Build history of the part. All positions in model axes, mm. Face numbers are marked on the shaded views. A direction names the side the tool comes from. Give positions to 0.01 mm unless a question says otherwise; leave off trailing zeros. Loops run counter-clockwise (first coordinate to the right, second up) from the corner with the lowest first, then second, coordinate; pieces in that order, holes last. Notation, with made-up numbers: (23, 67.25) - (51, 67.25) arc R5 ccw to (51, 75.25) - close; hole circle Ø9 at (-5.75, -37.75). An arc over 180 degrees is marked (long way). Return JSON: item names as keys, results as strings. Group by question number.
1) Slice it at C-C (y = -31.5). List the corners of the cut face in (x, z), and give its area (3 significant figures).
2) Drop flat-ended pins along their axis: pin 1 (6 mm diameter, centred on y = 1.5, z = -58.5, fed in from +X); pin 2 (4 mm diameter, centred on x = 25.88, z = -96.59, fed in from +Y); pin 3 (4 mm diameter, centred on x = -9, y = 50.5, fed in from -Z). Give the stop position or say it passes through.
3) 3-axis set-ups, long thin cutter, end or side, ignore diameter. For the marked faces 1, 2 and 3: which of +Z, -Z, +X, -X, +Y, -Y reach the whole face in a straight line?
4) Drill centre lines: probe 1 along Y at (x, z) = (-102, -10.5); probe 2 along X at (y, z) = (19, -10); probe 3 along Y at (x, z) = (-52.5, -60). Where is each one in solid material? Low to high. Write a range as from..to.
5) Slice it at B-B (x = 0). List the corners of the cut face in (y, z).
6) Slice it at A-A (y = 19.8). List the corners of the cut face in (x, z).
7) Slice it at D-D (y = 68.5). List the corners of the cut face in (x, z).
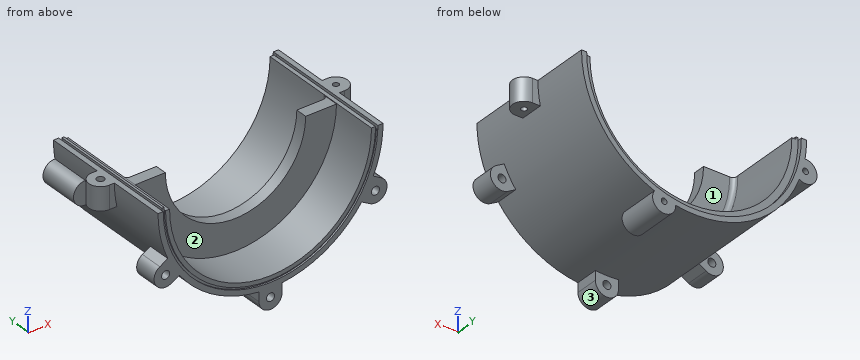
```python
from build123d import *

# Parameters (mm, degrees)
REVOLU_O2_ANGLE            = 180
ESBO_O4_R                  = 10
RESSALTO_EXTRUS_O1_DEPTH   = 35
RESSALTO_EXTRUS_O2_DEPTH   = 20
ESBO_O8_R                  = 3.5
CORTE_EXTRUS_O2_DEPTH      = 20
PADR_OCIRCULAR1_COUNT      = 6
ESBO_O6_R                  = 2.5
CORTE_EXTRUS_O1_DEPTH      = 15
ESBO_O10_W                 = 2.2
ESBO_O10_H                 = 116.4
CORTE_EXTRUS_O4_DEPTH      = 3.5
ESBO_O11_W                 = 2
ESBO_O11_H                 = 114.9
RESSALTO_EXTRUS_O5_DEPTH   = 2
ESBO_O12_R                 = 3.25
RESSALTO_EXTRUS_O6_DEPTH   = 20
ESBO_O13_R                 = 2.5
RESSALTO_EXTRUS_O7_DEPTH   = 20
ESBO_O16_R                 = 93
CORTE_EXTRUS_O6_DEPTH      = 10
ESBO_O17_R                 = 92.967356783
ESBO_O17_R_2               = 90.967356783
CORTE_EXTRUS_O7_DEPTH      = 1.5
CORTE_EXTRUS_O9_DEPTH      = 41.2
CORTE_EXTRUS_O9_DEPTH_BACK = 80.8


with BuildPart() as part:
    # Esboço3 → Revolução2 (revolve)
    with BuildSketch(Plane.XY):
        with BuildLine():
            Line((97.5, 79.8), (97.5, 11.304491341))
            Line((97.5, 11.304491341), (97.5, 0))
            Line((97.5, 0), (97.5, -40.2))
            Line((97.5, -40.2), (87.5, -40.2))
            Line((87.5, -40.2), (87.5, 0))
            Line((87.5, 0), (60.342408243, 0))
            Line((60.342408243, 0), (60.342408243, 10.2))
            Line((60.342408243, 10.2), (83.5, 10.2))
            ThreePointArc((83.5, 10.2), (86.328427125, 11.371572875), (87.5, 14.2))
            Line((87.5, 14.2), (87.5, 76.2))
            Line((87.5, 76.2), (93, 76.2))
            Line((93, 76.2), (93, 79.8))
            Line((93, 79.8), (97.5, 79.8))
        make_face()
    revolve(axis=Axis((0, -3.322055656, 0), (0, 1, 0)), revolution_arc=REVOLU_O2_ANGLE)

    # Esboço4 → Ressalto-extrusão1 (add)
    with BuildSketch(Plane(origin=(0, 79.8, 0), x_dir=(1, 0, 0), z_dir=(0, 1, 0))):
        with Locations((25.881656302, 96.591656302)):
            Circle(ESBO_O4_R)
        with Locations((-96.591656302, 25.881656302)):
            Circle(ESBO_O4_R)
    extrude(amount=-RESSALTO_EXTRUS_O1_DEPTH)

    # Esboço5 → Ressalto-extrusão2 (add)
    with BuildSketch(Plane.XZ.offset(40.2)):
        with BuildLine():
            Line((10, -105), (10, -96.985823706))
            Line((10, -96.985823706), (-10, -96.985823706))
            Line((-10, -96.985823706), (-10, -105))
            ThreePointArc((-10, -105), (0, -115), (10, -105))
        make_face()
    ressalto_extrus_o2 = extrude(amount=-RESSALTO_EXTRUS_O2_DEPTH)

    # Esboço8 → Corte-extrusão2 (cut)
    with BuildSketch(Plane.XZ.offset(40.2)):
        with Locations((0, -105)):
            Circle(ESBO_O8_R)
    corte_extrus_o2 = extrude(amount=-CORTE_EXTRUS_O2_DEPTH, mode=Mode.SUBTRACT)

    # PadrãoCircular1: Ressalto-extrusão2, Corte-extrusão2 ×6 about axis, 3 skipped
    padr_ocircular1_axis = Axis((0, 0, 0), (0, 1, 0))
    add([ressalto_extrus_o2.rotate(padr_ocircular1_axis, i * 360 / PADR_OCIRCULAR1_COUNT) for i in range(1, PADR_OCIRCULAR1_COUNT) if i not in (2, 3, 4)])
    add([corte_extrus_o2.rotate(padr_ocircular1_axis, i * 360 / PADR_OCIRCULAR1_COUNT) for i in range(1, PADR_OCIRCULAR1_COUNT) if i not in (2, 3, 4)], mode=Mode.SUBTRACT)

    # Esboço6 → Corte-extrusão1 (cut)
    with BuildSketch(Plane(origin=(0, 79.8, 0), x_dir=(1, 0, 0), z_dir=(0, 1, 0))):
        with Locations((25.881656302, 96.591656302)):
            Circle(ESBO_O6_R)
        with Locations((-96.591656302, 25.881656302)):
            Circle(ESBO_O6_R)
    extrude(amount=-CORTE_EXTRUS_O1_DEPTH, mode=Mode.SUBTRACT)

    # Esboço10 → Corte-extrusão4 (cut)
    with BuildSketch(Plane.XY):
        with Locations((92, 18)):
            Rectangle(ESBO_O10_W, ESBO_O10_H)
    extrude(amount=-CORTE_EXTRUS_O4_DEPTH, mode=Mode.SUBTRACT)

    # Esboço11 → Ressalto-extrusão5 (add)
    with BuildSketch(Plane.XY):
        with Locations((-92, 18.75)):
            Rectangle(ESBO_O11_W, ESBO_O11_H)
    extrude(amount=RESSALTO_EXTRUS_O5_DEPTH)

    # Esboço12 → Ressalto-extrusão6 (add)
    with BuildSketch(Plane.XY):
        with BuildLine():
            Line((-102, 29.8), (-87.5, 29.8))
            Line((-87.5, 29.8), (-87.5, 9.8))
            Line((-87.5, 9.8), (-102, 9.8))
            ThreePointArc((-102, 9.8), (-112, 19.8), (-102, 29.8))
        make_face()
        with Locations((-102, 19.8)):
            Circle(ESBO_O12_R, mode=Mode.SUBTRACT)
    extrude(amount=-RESSALTO_EXTRUS_O6_DEPTH)

    # Esboço13 → Ressalto-extrusão7 (add)
    with BuildSketch(Plane.XY):
        with BuildLine():
            Line((102, 29.8), (93.1, 29.8))
            Line((93.1, 29.8), (93.1, 9.8))
            Line((93.1, 9.8), (102, 9.8))
            ThreePointArc((102, 9.8), (112, 19.8), (102, 29.8))
        make_face()
        with Locations((102, 19.8)):
            Circle(ESBO_O13_R, mode=Mode.SUBTRACT)
    extrude(amount=-RESSALTO_EXTRUS_O7_DEPTH)

    # Esboço16 → Corte-extrusão6 (cut)
    with BuildSketch(Plane(origin=(0, 76.2, 0), x_dir=(1, 0, 0), z_dir=(0, 1, 0))):
        Circle(ESBO_O16_R)
    extrude(amount=CORTE_EXTRUS_O6_DEPTH, mode=Mode.SUBTRACT)

    # Esboço17 → Corte-extrusão7 (cut)
    with BuildSketch(Plane.XZ.offset(40.2)):
        Circle(ESBO_O17_R)
        Circle(ESBO_O17_R_2, mode=Mode.SUBTRACT)
    extrude(amount=-CORTE_EXTRUS_O7_DEPTH, mode=Mode.SUBTRACT)

    # Esboço21 → Corte-extrusão9 (cut, two sides)
    with BuildSketch(Plane.XZ) as corte_extrus_o9_sk:
        with BuildLine():
            Line((-87.5, 0), (87.5, 0))
            ThreePointArc((87.5, 0), (87.499642853, -0.25000102), (87.498571417, -0.5))
            Line((87.498571417, -0.5), (60.84035372, -0.5))
            ThreePointArc((60.84035372, -0.5), (0, -60.842408243), (-60.84035372, -0.5))
            Line((-60.84035372, -0.5), (-87.498571417, -0.5))
            ThreePointArc((-87.498571417, -0.5), (-87.499642853, -0.25000102), (-87.5, 0))
        make_face()
    extrude(amount=CORTE_EXTRUS_O9_DEPTH, mode=Mode.SUBTRACT)
    extrude(corte_extrus_o9_sk.sketch, amount=-CORTE_EXTRUS_O9_DEPTH_BACK, mode=Mode.SUBTRACT)


solid = part.part
```
Results:
{
 "1": {"outline": "(-97.5, 0) arc R97.5 ccw to (-88.99, -39.83) - (-95.93, -43.84) arc R10 ccw to (-85.93, -61.16) - (-78.99, -57.15) arc R97.5 ccw to (-10, -96.99) - (-10, -105) arc R10 ccw to (10, -105) - (10, -96.99) arc R97.5 ccw to (78.99, -57.15) - (85.93, -61.16) arc R10 ccw to (95.93, -43.84) - (88.99, -39.83) arc R97.5 ccw to (97.5, 0) - (93.1, 0) - (93.1, -3.5) - (90.9, -3.5) - (90.9, 0) - (87.5, 0) arc R87.5 cw to (-87.5, 0) - (-91, 0) - (-91, 2) - (-93, 2) - (-93, 0) - close; hole circle Ø7 at (-90.93, -52.5); hole circle Ø7 at (0, -105); hole circle Ø7 at (90.93, -52.5)", "area": "3,720 mm2"},
 "2": {"pin 1": "x = 80.16", "pin 2": "y = 64.8", "pin 3": "z = -97.25"},
 "3": {"face 1": "+Z, +Y", "face 2": "+Z, -Y", "face 3": "-Z, +Y, -Y"},
 "4": {"probe 1": "9.8..16.55, 23.05..29.8", "probe 2": "-111.97..-105.15, -98.85..-86.93, 86.93..99.63, 104.37..111.97", "probe 3": "0..10.2"},
 "5": {"outline": "(-40.2, -115) - (-20.2, -115) - (-20.2, -108.5) - (-40.2, -108.5) - close; (-40.2, -101.5) - (-20.2, -101.5) - (-20.2, -97.5) - (79.8, -97.5) - (79.8, -93) - (76.2, -93) - (76.2, -87.5) - (14.2, -87.5) arc R4 cw to (10.2, -83.5) - (10.2, -60.84) - (0, -60.84) - (0, -87.5) - (-40.2, -87.5) - (-40.2, -90.97) - (-38.7, -90.97) - (-38.7, -92.97) - (-40.2, -92.97) - close"},
 "6": {"outline": "(-112, -20) - (-105.25, -20) - (-105.25, 0) - (-112, 0) - close; (-98.75, -20) - (-95.43, -20) arc R97.5 ccw to (95.43, -20) - (99.5, -20) - (99.5, 0) - (93.1, 0) - (93.1, -3.5) - (90.9, -3.5) - (90.9, 0) - (87.5, 0) arc R87.5 cw to (-87.5, 0) - (-91, 0) - (-91, 2) - (-93, 2) - (-93, 0) - (-98.75, 0) - close; (104.5, -20) - (112, -20) - (112, 0) - (104.5, 0) - close"},
 "7": {"outline": "(-97.5, 0) arc R97.5 ccw to (-96.2, -15.89) arc R10 ccw (long way) to (-91.25, -34.34) arc R97.5 ccw to (15.89, -96.2) arc R10 ccw (long way) to (34.34, -91.25) arc R97.5 ccw to (97.5, 0) - (93.1, 0) - (93.1, -3.5) - (90.9, -3.5) - (90.9, 0) - (87.5, 0) arc R87.5 cw to (-87.5, 0) - (-91, 0) - (-91, 2) - (-93, 2) - (-93, 0) - close; hole circle Ø5 at (-96.59, -25.88); hole circle Ø5 at (25.88, -96.59)"}
}
